Here's how the part is built. I have some questions about the finished solid (model axes, mm). Face numbers are marked on the shaded views. A direction names the side the tool comes from. Give positions to 0.01 mm unless a question says otherwise; leave off trailing zeros. Loops run counter-clockwise (first coordinate to the right, second up) from the corner with the lowest first, then second, coordinate; pieces in that order, holes last. Notation, with made-up numbers: (76, 58) - (84, 58) arc R21 cw to (84, 91) - close; hole circle Ø5 at (-25.5, -25). An arc over 180 degrees is marked (long way). Use one line per item in the form item = value.
Autodesk Inventor part; units mm, degrees
ref_plane "center_point_XY" through (4, 0, 0) normal (1, 0, 0) x (0, 0, -1)
ref_plane "center_point_YZ" through (4, 0, 0) normal (0, 0, -1) x (0, 1, 0)
ref_plane "center_point_ZX" through (4, 0, 0) normal (0, 1, 0) x (1, 0, 0)
sketch "Sketch_1" plane through (0, 0, 0) normal (0, 0, 1) x (1, 0, 0)
  line L0 (8, 0) -> (0, 0)
  arc A0 (0, 5.3) -> (0.3, 5) centre (0.3, 5.3) ccw
  line L1 (0.3, 5) -> (7.7, 5)
  arc A1 (7.7, 5) -> (8, 5.3) centre (7.7, 5.3) ccw
  line L2 (8, 5.3) -> (8, 6.95)
  line L3 (8, 6.95) -> (7.669, 6.95)
  line L4 (7.669, 6.95) -> (7.669, 11.1)
  line L5 (7.669, 11.1) -> (8, 11.1)
  line L6 (8, 11.1) -> (8, 12.7)
  arc A2 (8, 12.7) -> (7.7, 13) centre (7.7, 12.7) ccw
  line L7 (7.7, 13) -> (0.3, 13)
  arc A3 (0.3, 13) -> (0, 12.7) centre (0.3, 12.7) ccw
  line L8 (0, 12.7) -> (0, 11.1)
  line L9 (0, 11.1) -> (0.331, 11.1)
  line L10 (0.331, 11.1) -> (0.331, 6.95)
  line L11 (0.331, 6.95) -> (0, 6.95)
  line L12 (0, 6.95) -> (0, 5.3)
revolve "Revolution1" add sketch "Sketch_1" angle 360 about axis through (8, 0, 0) along (1, 0, 0)
ref_plane "center_point_XY" through (4, 0, 0) normal (1, 0, 0) x (0, 0, -1)
ref_plane "center_point_YZ" through (4, 0, 0) normal (0, 0, -1) x (0, 1, 0)
ref_plane "center_point_ZX" through (4, 0, 0) normal (0, 1, 0) x (1, 0, 0)
ref_plane "to_housing_XY" through (0, 0, 0) normal (1, 0, 0) x (0, 0, -1)
ref_plane "to_housing_YZ" through (0, 0, 0) normal (0, 0, -1) x (0, 1, 0)
ref_plane "to_housing_ZX" through (0, 0, 0) normal (0, 1, 0) x (1, 0, 0)
ref_plane "to_ring_XY" through (7.338, 0, 0) normal (1, 0, 0) x (0, 0, -1)
ref_plane "to_ring_YZ" through (7.338, 0, 0) normal (0, 0, -1) x (0, 1, 0)
ref_plane "to_ring_ZX" through (7.338, 0, 0) normal (0, 1, 0) x (1, 0, 0)
properties part number "bearing_6000"
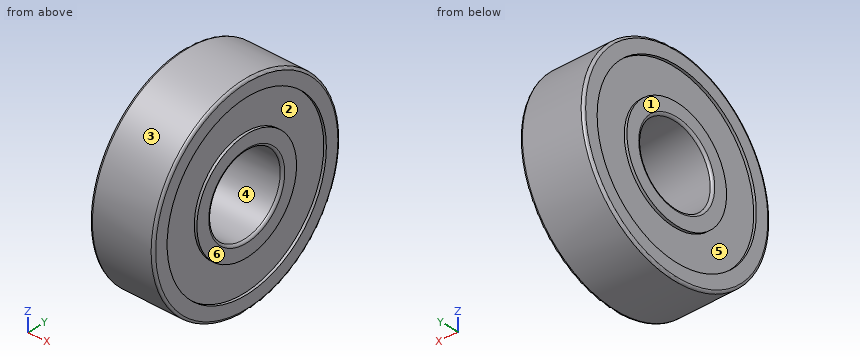
(1) For P1, Ø1, axis at y = -3.5, z = 8, coming from the -X side; P2, Ø4, axis at x = 4, y = -8.5, coming from the -Z side; P3, Ø2, axis at x = 3.5, y = 8, coming from the +Z side, each with a flat end and sliding along its axis, tell me the tip position at first contact or that it passes through.
Geometry says:
P1 = 0.33
P2 = -11.26
P3 = 10.95
(2) Thinking about a two-plate mould opening in Z: for the marked faces 3, 4, 5 and 6, which applies, pulls with the +Z half, pulls with the -Z half, needs draft (parallel to the pull), parting line crosses it, or undercut?
Geometry says:
face_3 = parting line crosses it
face_4 = undercut
face_5 = undercut
face_6 = needs draft
(3) If we section it at C-C (x = 6): List the corners of the cut face in (y, z) for me.
Geometry says:
outline = circle Ø26 at (0, 0); hole circle Ø10 at (0, 0)
(4) For the marked faces 1 and 2, which set-ups out of +Z, -Z, +X, -X, +Y, -Y let a thin tool reach every point of the face, with its end or its side?
Geometry says:
face_1 = +Z, -Z, -X, +Y, -Y
face_2 = +X
(5) If I drill on probe 1 along Z at (x, y) = (0.25, 0); probe 2 along Z at (x, y) = (4.75, 0); probe 3 along Z at (x, y) = (6.5, -4), over which ranges is the centre line in solid material (lowest first)?
Geometry says:
probe_1 = -13 to -11.1, -6.95 to -5, 5 to 6.95, 11.1 to 13
probe_2 = -13 to -5, 5 to 13
probe_3 = -12.37 to -3, 3 to 12.37
